from build123d import *

# Parameters (mm, degrees)
CYLINDER776_R                = 1.5
CYLINDER776_DEPTH            = 20
CYLINDER774_R                = 1.5
CYLINDER774_DEPTH            = 20
COMPOUND536_ROLL_ANGLE       = 90
COMPOUND536_PLACEMENT_ANGLE  = 90
BOX640_W                     = 16
BOX640_H                     = 8
BOX640_DEPTH                 = 3
BOX639_W                     = 16
BOX639_H                     = 8
BOX639_DEPTH                 = 3
BOX636_W                     = 16
BOX636_H                     = 8
BOX636_DEPTH                 = 3
BOX637_W                     = 16
BOX637_H                     = 8
BOX637_DEPTH                 = 3
CYLINDER1600_R               = 12
CYLINDER1600_DEPTH           = 20
CYLINDER1598_R               = 5
CYLINDER1598_DEPTH           = 4
CYLINDER1605_R               = 5
CYLINDER1605_DEPTH           = 4
CYLINDER1612_R               = 5
CYLINDER1612_DEPTH           = 4
CYLINDER1610_R               = 5
CYLINDER1610_DEPTH           = 4
CYLINDER1604_R               = 2.5
CYLINDER1604_DEPTH           = 20
CYLINDER1608_R               = 2.5
CYLINDER1608_DEPTH           = 20
CYLINDER1607_R               = 2.5
CYLINDER1607_DEPTH           = 20
CYLINDER1602_R               = 2.5
CYLINDER1602_DEPTH           = 20
CYLINDER1609_R               = 3
CYLINDER1609_DEPTH           = 3
CYLINDER1609_PLACEMENT_ANGLE = 22.5
CYLINDER1601_R               = 3
CYLINDER1601_DEPTH           = 3
CYLINDER1601_PLACEMENT_ANGLE = 67.5
CYLINDER1606_R               = 3
CYLINDER1606_DEPTH           = 3
CYLINDER1606_PLACEMENT_ANGLE = 202.5
CYLINDER1611_R               = 3
CYLINDER1611_DEPTH           = 3
CYLINDER1611_PLACEMENT_ANGLE = 112.5
COMPOUND801_PLACEMENT_ANGLE  = 45
CYLINDER1603_R               = 1.5
CYLINDER1603_DEPTH           = 30
CYLINDER1603_PLACEMENT_ANGLE = 22.5
CYLINDER1613_R               = 1.5
CYLINDER1613_DEPTH           = 30
CYLINDER1613_PLACEMENT_ANGLE = 67.5
CYLINDER1614_R               = 1.5
CYLINDER1614_DEPTH           = 30
CYLINDER1614_PLACEMENT_ANGLE = 202.5
CYLINDER1599_R               = 1.5
CYLINDER1599_DEPTH           = 30
CYLINDER1599_PLACEMENT_ANGLE = 112.5
COMPOUND802_PLACEMENT_ANGLE  = 45
BOX638_W                     = 64
BOX638_H                     = 64
BOX638_DEPTH                 = 8


with BuildPart() as obj1:
    # Cylinder776 → Cylinder776 (new body)
    with BuildSketch(Plane(origin=(15.75, 114, 59.48), x_dir=(-1, 0, 0), z_dir=(0, 1, 0))):
        Circle(CYLINDER776_R)
    extrude(amount=CYLINDER776_DEPTH)


with BuildPart() as compound536:
    # Cylinder774 → Cylinder774 (new body)
    with BuildSketch(Plane(origin=(15.75, 114, 38.52), x_dir=(-1, 0, 0), z_dir=(0, 1, 0))):
        Circle(CYLINDER774_R)
    extrude(amount=CYLINDER774_DEPTH)

    # Compound536: union obj1
    add(obj1.part)


with BuildPart() as compound536_1:
    # Compound536 roll: moved
    add(compound536.part.rotate(Axis((0, 0, 0), (1, 0, 0)), COMPOUND536_ROLL_ANGLE))


with BuildPart() as compound536_2:
    # Compound536 placement: moved
    add(compound536_1.part.moved(Location((-49, 0, -96))).rotate(Axis((-49, 0, -96), (0, 0, 1)), COMPOUND536_PLACEMENT_ANGLE))


with BuildPart() as krychle640:
    # Box640 → Box640 (new body)
    with BuildSketch(Plane(origin=(17.55, -27.55, 31), x_dir=(1, 0, 0), z_dir=(0, 0, 1))):
        with Locations((8, 4)):
            Rectangle(BOX640_W, BOX640_H)
    extrude(amount=BOX640_DEPTH)


with BuildPart() as krychle639:
    # Box639 → Box639 (new body)
    with BuildSketch(Plane(origin=(-33.45, 19.55, 31), x_dir=(1, 0, 0), z_dir=(0, 0, 1))):
        with Locations((8, 4)):
            Rectangle(BOX639_W, BOX639_H)
    extrude(amount=BOX639_DEPTH)


with BuildPart() as krychle636:
    # Box636 → Box636 (new body)
    with BuildSketch(Plane(origin=(-33.45, -27.55, 31), x_dir=(1, 0, 0), z_dir=(0, 0, 1))):
        with Locations((8, 4)):
            Rectangle(BOX636_W, BOX636_H)
    extrude(amount=BOX636_DEPTH)


with BuildPart() as compound800:
    # Box637 → Box637 (new body)
    with BuildSketch(Plane(origin=(17.55, 19.55, 31), x_dir=(1, 0, 0), z_dir=(0, 0, 1))):
        with Locations((8, 4)):
            Rectangle(BOX637_W, BOX637_H)
    extrude(amount=BOX637_DEPTH)

    # Compound800: union Krychle640, Krychle639, Krychle636
    add(krychle640.part)
    add(krychle639.part)
    add(krychle636.part)


with BuildPart() as obj2:
    # Cylinder1600 → Cylinder1600 (new body)
    with BuildSketch(Plane.XY.offset(15)):
        Circle(CYLINDER1600_R)
    extrude(amount=CYLINDER1600_DEPTH)


with BuildPart() as obj3:
    # Cylinder1598 → Cylinder1598 (new body)
    with BuildSketch(Plane(origin=(23.55, 23.55, 26), x_dir=(1, 0, 0), z_dir=(0, 0, 1))):
        Circle(CYLINDER1598_R)
    extrude(amount=CYLINDER1598_DEPTH)


with BuildPart() as obj4:
    # Cylinder1605 → Cylinder1605 (new body)
    with BuildSketch(Plane(origin=(23.55, -23.55, 26), x_dir=(1, 0, 0), z_dir=(0, 0, 1))):
        Circle(CYLINDER1605_R)
    extrude(amount=CYLINDER1605_DEPTH)


with BuildPart() as obj5:
    # Cylinder1612 → Cylinder1612 (new body)
    with BuildSketch(Plane(origin=(-23.55, 23.55, 26), x_dir=(1, 0, 0), z_dir=(0, 0, 1))):
        Circle(CYLINDER1612_R)
    extrude(amount=CYLINDER1612_DEPTH)


with BuildPart() as compound799:
    # Cylinder1610 → Cylinder1610 (new body)
    with BuildSketch(Plane(origin=(-23.55, -23.55, 26), x_dir=(1, 0, 0), z_dir=(0, 0, 1))):
        Circle(CYLINDER1610_R)
    extrude(amount=CYLINDER1610_DEPTH)

    # Compound799: union obj3, obj4, obj5
    add(obj3.part)
    add(obj4.part)
    add(obj5.part)


with BuildPart() as compound799_1:
    # Compound799 placement: moved
    add(compound799.part.moved(Location((0, 0, -50))))


with BuildPart() as obj6:
    # Cylinder1604 → Cylinder1604 (new body)
    with BuildSketch(Plane(origin=(-23.55, 23.55, 20), x_dir=(1, 0, 0), z_dir=(0, 0, 1))):
        Circle(CYLINDER1604_R)
    extrude(amount=CYLINDER1604_DEPTH)


with BuildPart() as obj7:
    # Cylinder1608 → Cylinder1608 (new body)
    with BuildSketch(Plane(origin=(-23.55, -23.55, 20), x_dir=(1, 0, 0), z_dir=(0, 0, 1))):
        Circle(CYLINDER1608_R)
    extrude(amount=CYLINDER1608_DEPTH)


with BuildPart() as obj8:
    # Cylinder1607 → Cylinder1607 (new body)
    with BuildSketch(Plane(origin=(23.55, -23.55, 20), x_dir=(1, 0, 0), z_dir=(0, 0, 1))):
        Circle(CYLINDER1607_R)
    extrude(amount=CYLINDER1607_DEPTH)


with BuildPart() as compound798:
    # Cylinder1602 → Cylinder1602 (new body)
    with BuildSketch(Plane(origin=(23.55, 23.55, 20), x_dir=(1, 0, 0), z_dir=(0, 0, 1))):
        Circle(CYLINDER1602_R)
    extrude(amount=CYLINDER1602_DEPTH)

    # Compound798: union obj6, obj7, obj8
    add(obj6.part)
    add(obj7.part)
    add(obj8.part)


with BuildPart() as obj9:
    # Cylinder1609 → Cylinder1609 (new body)
    with BuildSketch(Plane.XY):
        Circle(CYLINDER1609_R)
    extrude(amount=CYLINDER1609_DEPTH)


with BuildPart() as obj9_1:
    # Cylinder1609 placement: moved
    add(obj9.part.moved(Location((-16, 0, 2))).rotate(Axis((-16, 0, 2), (0, 0, 1)), CYLINDER1609_PLACEMENT_ANGLE))


with BuildPart() as obj10:
    # Cylinder1601 → Cylinder1601 (new body)
    with BuildSketch(Plane.XY):
        Circle(CYLINDER1601_R)
    extrude(amount=CYLINDER1601_DEPTH)


with BuildPart() as obj10_1:
    # Cylinder1601 placement: moved
    add(obj10.part.moved(Location((0, 16, 2))).rotate(Axis((0, 16, 2), (0, 0, -1)), CYLINDER1601_PLACEMENT_ANGLE))


with BuildPart() as obj11:
    # Cylinder1606 → Cylinder1606 (new body)
    with BuildSketch(Plane.XY):
        Circle(CYLINDER1606_R)
    extrude(amount=CYLINDER1606_DEPTH)


with BuildPart() as obj11_1:
    # Cylinder1606 placement: moved
    add(obj11.part.moved(Location((16, 0, 2))).rotate(Axis((16, 0, 2), (0, 0, 1)), CYLINDER1606_PLACEMENT_ANGLE))


with BuildPart() as compound801:
    # Cylinder1611 → Cylinder1611 (new body)
    with BuildSketch(Plane.XY):
        Circle(CYLINDER1611_R)
    extrude(amount=CYLINDER1611_DEPTH)


with BuildPart() as compound801_1:
    # Cylinder1611 placement: moved
    add(compound801.part.moved(Location((0, -16, 2))).rotate(Axis((0, -16, 2), (0, 0, 1)), CYLINDER1611_PLACEMENT_ANGLE))

    # Compound801: union obj9, obj10, obj11
    add(obj9_1.part)
    add(obj10_1.part)
    add(obj11_1.part)


with BuildPart() as compound801_2:
    # Compound801 placement: moved
    add(compound801_1.part.moved(Location((0, 0, 29))).rotate(Axis((0, 0, 29), (0, 0, 1)), COMPOUND801_PLACEMENT_ANGLE))


with BuildPart() as obj12:
    # Cylinder1603 → Cylinder1603 (new body)
    with BuildSketch(Plane.XY):
        Circle(CYLINDER1603_R)
    extrude(amount=CYLINDER1603_DEPTH)


with BuildPart() as obj12_1:
    # Cylinder1603 placement: moved
    add(obj12.part.moved(Location((-16, 0, 2))).rotate(Axis((-16, 0, 2), (0, 0, 1)), CYLINDER1603_PLACEMENT_ANGLE))


with BuildPart() as obj13:
    # Cylinder1613 → Cylinder1613 (new body)
    with BuildSketch(Plane.XY):
        Circle(CYLINDER1613_R)
    extrude(amount=CYLINDER1613_DEPTH)


with BuildPart() as obj13_1:
    # Cylinder1613 placement: moved
    add(obj13.part.moved(Location((0, 16, 2))).rotate(Axis((0, 16, 2), (0, 0, -1)), CYLINDER1613_PLACEMENT_ANGLE))


with BuildPart() as obj14:
    # Cylinder1614 → Cylinder1614 (new body)
    with BuildSketch(Plane.XY):
        Circle(CYLINDER1614_R)
    extrude(amount=CYLINDER1614_DEPTH)


with BuildPart() as obj14_1:
    # Cylinder1614 placement: moved
    add(obj14.part.moved(Location((16, 0, 2))).rotate(Axis((16, 0, 2), (0, 0, 1)), CYLINDER1614_PLACEMENT_ANGLE))


with BuildPart() as compound802:
    # Cylinder1599 → Cylinder1599 (new body)
    with BuildSketch(Plane.XY):
        Circle(CYLINDER1599_R)
    extrude(amount=CYLINDER1599_DEPTH)


with BuildPart() as compound802_1:
    # Cylinder1599 placement: moved
    add(compound802.part.moved(Location((0, -16, 2))).rotate(Axis((0, -16, 2), (0, 0, 1)), CYLINDER1599_PLACEMENT_ANGLE))

    # Compound802: union obj12, obj13, obj14
    add(obj12_1.part)
    add(obj13_1.part)
    add(obj14_1.part)


with BuildPart() as compound802_2:
    # Compound802 placement: moved
    add(compound802_1.part.moved(Location((0, 0, 14))).rotate(Axis((0, 0, 14), (0, 0, 1)), COMPOUND802_PLACEMENT_ANGLE))


with BuildPart() as cut179:
    # Box638 → Box638 (new body)
    with BuildSketch(Plane(origin=(-32, -32, 26), x_dir=(1, 0, 0), z_dir=(0, 0, 1))):
        with Locations((32, 32)):
            Rectangle(BOX638_W, BOX638_H)
    extrude(amount=BOX638_DEPTH)

    # Cut173: cut Compound802
    add(compound802_2.part, mode=Mode.SUBTRACT)

    # Cut174: cut Compound801
    add(compound801_2.part, mode=Mode.SUBTRACT)

    # Cut177: cut Compound798
    add(compound798.part, mode=Mode.SUBTRACT)

    # Cut175: cut Compound799
    add(compound799_1.part, mode=Mode.SUBTRACT)

    # Cut176: cut obj2
    add(obj2.part, mode=Mode.SUBTRACT)

    # Cut178: cut Compound800
    add(compound800.part, mode=Mode.SUBTRACT)

    # Cut179: cut Compound536
    add(compound536_2.part, mode=Mode.SUBTRACT)


solid = cut179.part
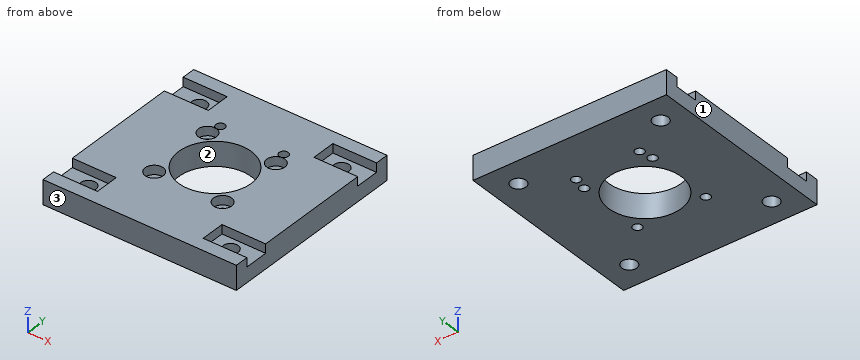
Verification items for the finished model (mm, model axes). Face numbers are marked on the shaded views. Coordinates: 2 decimals unless noted, no trailing zeros. Order: outer loops, then holes, each group sorted by start corner. A loop starts at its lowest first (then second) coordinate and runs counter-clockwise, first axis right, second up. Notation, with made-up numbers: M -14.5,47.5 L 2.5,47.5 A6 cw 2.5,52.5 Z; hole C 77.25,22 d5. An arc over 180 degrees is marked long. One line per item, written item: value. Start each with the question number.
Item 1: Sectioned sample at D-D on z = 33. Record the cut outline in (x, y), then the cut area to 3 significant figures.
Item 2: Sectioned sample at B-B on x = -23.55. Record the cut outline in (y, z), then the cut area to 3 significant figures.
Item 3: Thickness scan on probe 1 along X at (y, z) = (-23.5, 28); probe 2 along Y at (x, z) = (28.5, 32.25). Record the ranges inside material, lowest first.
Item 4: Sectioned sample at A-A on y = 0. Record the cut outline in (x, z), then the cut area to 3 significant figures.
Item 5: Depth check by flat-ended pin: P1, Ø2.5, axis at x = -11.31, y = -11.31, coming from the +Z side; P2, Ø5, axis at x = 11.31, y = -11.31, coming from the +Z side; P3, Ø1.5, axis at y = 24.5, z = 32.5, coming from the +X side. Enter the tip coordinate at first touch or a pass-through.
Item 6: Mould release check, pull along X, two halves, no side actions. Record for the marked faces 1, 2 and 3: pulls with the +X half, pulls with the -X half, needs draft (parallel to the pull), parting line crosses it, or undercut.
Calculated:
1. outline: M -32,-32 L 32,-32 L 32,-27.55 L 17.55,-27.55 L 17.55,-19.55 L 32,-19.55 L 32,19.55 L 17.55,19.55 L 17.55,27.55 L 32,27.55 L 32,32 L -32,32 L -32,27.55 L -17.45,27.55 L -17.45,19.55 L -32,19.55 L -32,-19.55 L -17.45,-19.55 L -17.45,-27.55 L -32,-27.55 Z; hole C -11.31,-11.31 d6; hole C -11.31,11.31 d6; hole C 0,0 d24; hole C -10.48,15.75 d3; hole C 11.31,-11.31 d6; hole C 11.31,11.31 d6; hole C 10.48,15.75 d3
1. area: 3,050 mm^2
2. outline: M -32,26 L -26.05,26 L -26.05,31 L -27.55,31 L -27.55,34 L -32,34 Z; M -21.05,26 L 21.05,26 L 21.05,31 L 19.55,31 L 19.55,34 L -19.55,34 L -19.55,31 L -21.05,31 Z; M 26.05,26 L 32,26 L 32,34 L 27.55,34 L 27.55,31 L 26.05,31 Z
2. area: 414 mm^2
3. probe 1: -32 to -26.05, -21.05 to 21.05, 26.05 to 32
3. probe 2: -32 to -27.55, -19.55 to 19.55, 27.55 to 32
4. outline: M -32,26 L -12,26 L -12,34 L -32,34 Z; M 12,26 L 32,26 L 32,34 L 12,34 Z
4. area: 320 mm^2
5. P1: through
5. P2: z = 31
5. P3: x = 17.55
6. face 1: pulls with the -X half
6. face 2: undercut
6. face 3: needs draft
